Autodesk Inventor part; units mm, degrees
ref_plane "YZ Plane" through (0, 0, 0) normal (1, 0, 0) x (0, 1, 0)
ref_plane "XZ Plane" through (0, 0, 0) normal (0, 1, 0) x (-1, 0, 0)
ref_plane "XY Plane" through (0, 0, 0) normal (0, 0, 1) x (1, 0, 0)
sketch "Sketch1" plane through (0, 0, 0) normal (0, 1, 0) x (-1, 0, 0)
  line L0 (14, 13.5) -> (-14, 13.5)
  line L1 (-14, 13.5) -> (-14, -13.5)
  line L2 (-14, -13.5) -> (14, -13.5)
  line L3 (14, -13.5) -> (14, 13.5)
  line L4 (14, 13.5) -> (-14, -13.5) construction
  line L5 (-14, 13.5) -> (14, -13.5) construction
  line L6 (12.5, 12) -> (-12.5, 12)
  line L7 (-12.5, 12) -> (-12.5, -12)
  line L8 (-12.5, -12) -> (12.5, -12)
  line L9 (12.5, -12) -> (12.5, 12)
  point P0 (0, 0)
  dimension "d0" = 28
  dimension "d1" = 27
  dimension "d2" = 1.5
extrude "Extrusion1" add sketch "Sketch1" against normal blind 1.5 contours L3 L2 L1 L0 | L9 L8 L7 L6
hole "Hole1" at (-12.5, 0, 12) at (-12.5, 0, -12) at (12.5, 0, -12) at (12.5, 0, 12) direction (0, -1, 0) diameter 2 end through all
sketch "Sketch2" plane through (0, 0, 0) normal (0, 1, 0) x (1, 0, 0)
  circle A0 centre (12.5, 12) radius 1 construction
  circle A1 centre (-12.5, -12) radius 1 construction
  circle A2 centre (-12.5, 12) radius 1 construction
  circle A3 centre (12.5, -12) radius 1 construction
  line L0 (14, -13.5) -> (14, 13.5) construction
  line L1 (14, 13.5) -> (-14, 13.5) construction
  line L2 (-14, 13.5) -> (-14, -13.5) construction
  line L3 (-14, -13.5) -> (14, -13.5) construction
  line L4 (-11.3162, -13.5) -> (11.3667, -13.5)
  line L5 (11.3667, -13.5) -> (11.3667, 13.5)
  line L6 (11.3667, 13.5) -> (-11.3162, 13.5)
  line L7 (-11.3162, 13.5) -> (-11.3162, -13.5)
  point P0 (0, 0)
extrude "Extrusion2" add sketch "Sketch2" along normal blind 1
sketch "Sketch3" plane through (0, -1.5, 0) normal (0, -1, 0) x (1, 0, 0)
  line L0 (-14, 6) -> (-12, 6)
  line L1 (-12, 6) -> (-12, -6)
  line L2 (-12, -6) -> (-14, -6)
  line L3 (-14, -6) -> (-14, 6)
  line L4 (-14, 6) -> (-12, -6) construction
  line L5 (-12, 6) -> (-14, -6) construction
  line L6 (-14, 13.5) -> (-14, -13.5)
  point P0 (0, 0)
  point P1 (-13, 0)
  point P2 (-14, 0)
  dimension "d14" = 2
  dimension "d15" = 12
extrude "Extrusion3" add sketch "Sketch3" along normal blind 9
properties part number "screen_footprint"
Source: CAD feature listing. Evaluate the final solid. Frame: model axes, mm. A direction names the side the tool comes from. Give positions to 0.01 mm unless a question says otherwise; leave off trailing zeros. Order: outer loops, then holes, each group sorted by start corner. A loop starts at its lowest first (then second) coordinate and runs counter-clockwise, first axis right, second up.
(1) Section query C-C (y = -1). Return the cut outline in (x, z).
(2) Pull-direction query (Z, two-part tool) for faces 1 (the face through (13.1, -0.8, 11.2)), 2 (the face through (-13, -6, -6)), 3 (the face through (14, -1, 0)); classes: +Z half, -Z half, draft (parallel to the pull), parting line (faces both ways), or undercut.
(3) Section query B-B (x = -12.5). Return the cut outline in (y, z).
(4) Material intervals for line 1 along Z through (x, y) = (12.5, -0.6); line 2 along X through (y, z) = (-0.9, 12); line 3 along Y through (x, z) = (5.25, -4.5), sorted ascending.
(5) Access query for faces 4 (the face through (-12, -6, 0)), 5 (the face through (13, 0, 0)), 6 (the face through (-11.316, 0.5, -0.2)), 7 (the face through (-13, -6, 6)). Directions: +Z, -Z, +X, -X, +Y, -Y. A direction counts if a zero-diameter tool reaches every point of the face in a straight line with its end or side. Return the directions, or none.
(6) Section query A-A (z = -12). Return the cut outline in (x, y), plus the area to 3 significant figures.
(7) Section query D-D (x = 12.5). Return the cut outline in (y, z).
(8) Contact query for flat-ended pins moving along their axis: P1, Ø0.6, axis at x = -12.5, y = -5, coming from the -Z side; P2, Ø0.8, axis at y = 0.5, z = 3.5, coming from the +X side; P3, Ø2, axis at x = -1.5, z = -7, coming from the -Y side; P4, Ø1.2, axis at x = -12.5, z = 12, coming from the +Y side. Output: stop coordinate, or through.
Outcome:
1. outline: (-14, -13.5) - (14, -13.5) - (14, 13.5) - (-14, 13.5) - close; hole circle Ø2 at (-12.5, -12); hole circle Ø2 at (-12.5, 12); hole circle Ø2 at (12.5, -12); hole circle Ø2 at (12.5, 12)
2. face 1: undercut
2. face 2: -Z half
2. face 3: draft
3. outline: (-10.5, -6) - (-1.5, -6) - (-1.5, -11) - (0, -11) - (0, 11) - (-1.5, 11) - (-1.5, 6) - (-10.5, 6) - close; (-1.5, -13.5) - (0, -13.5) - (0, -13) - (-1.5, -13) - close; (-1.5, 13) - (0, 13) - (0, 13.5) - (-1.5, 13.5) - close
4. line 1: z = -13.5 to -13, -11 to 11, 13 to 13.5
4. line 2: x = -14 to -13.5, -11.5 to 11.5, 13.5 to 14
4. line 3: y = -1.5 to 1
5. face 4: +Z, -Z, +X, -Y
5. face 5: +Z, -Z, +X, +Y
5. face 6: +Z, -Z, -X, +Y
5. face 7: +Z, +X, -X, -Y
6. outline: (-14, -1.5) - (-13.5, -1.5) - (-13.5, 0) - (-14, 0) - close; (-11.5, -1.5) - (11.5, -1.5) - (11.5, 0) - (11.37, 0) - (11.37, 1) - (-11.32, 1) - (-11.32, 0) - (-11.5, 0) - close; (13.5, -1.5) - (14, -1.5) - (14, 0) - (13.5, 0) - close
6. area: 58.7 mm2
7. outline: (-1.5, -13.5) - (0, -13.5) - (0, -13) - (-1.5, -13) - close; (-1.5, -11) - (0, -11) - (0, 11) - (-1.5, 11) - close; (-1.5, 13) - (0, 13) - (0, 13.5) - (-1.5, 13.5) - close
8. P1: stops at z = -6
8. P2: stops at x = 11.37
8. P3: stops at y = -1.5
8. P4: passes through
